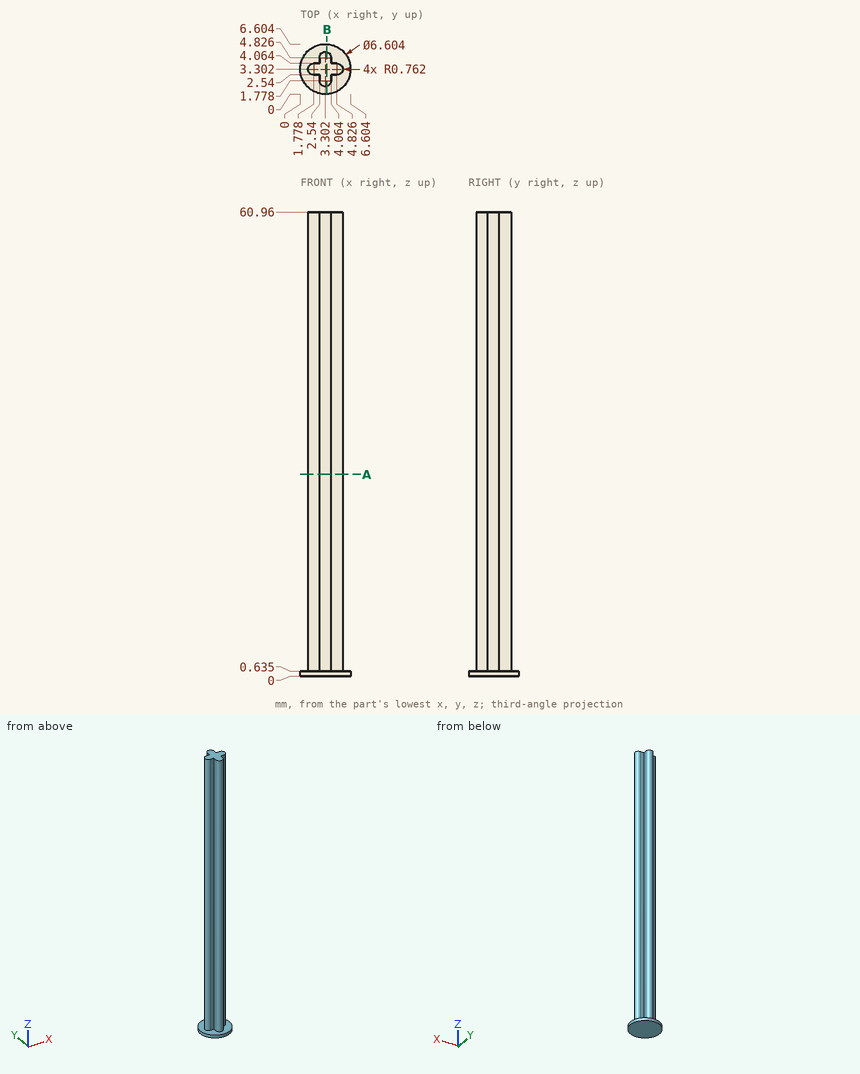
Input: dimensioned drawing with shaded views. Units: mm. Origin: part minimum x, y, z. Coordinates: 2 decimals unless noted, no trailing zeros. Loops run counter-clockwise (first coordinate to the right, second up) from the corner with the lowest first, then second, coordinate; pieces in that order, holes last. Notation, with made-up numbers: M 32,57.5 L 62,57.5 A24 cw 62,95.5 Z; hole C -6,66.5 d3. An arc over 180 degrees is marked long. Use a Markdown table: item, result. Add a question column.
1) Section A-A, the plane z = 26.5. Return the cut outline in (x, y), plus the area to 3 significant figures.
2) Pin query (flat end, axial travel): P1, Ø1.5, axis at y = 2, z = 33.5, coming from the -X side; P2, Ø3, axis at x = 2.5, z = 19, coming from the +Y side; P3, Ø0.6, axis at x = 2, z = 42, coming from the -Y side. Return the tip coordinate at first contact, or that it passes through.
3) Line query: L1, parallel to Z at x = 4.25, y = 0.5 (3 decimals); L2, parallel to Y at x = 2.25, z = 22. Output: solid intervals per line, ascending. Write a range as from..to.
4) Section B-B, the plane x = 3.5. Return the cut outline in (y, z) (3 decimals).
Answer below:
| question | item | result |
|---|---|---|
| 1 | outline | M 1.78,2.54 L 2.54,2.54 L 2.54,1.78 A0.76 ccw 4.06,1.78 L 4.06,2.54 L 4.83,2.54 A0.76 ccw 4.83,4.06 L 4.06,4.06 L 4.06,4.83 A0.76 ccw 2.54,4.83 L 2.54,4.06 L 1.78,4.06 A0.76 ccw Z |
| 1 | area | 10.6 mm2 |
| 2 | P1 | x = 1.25 |
| 2 | P2 | y = 5.59 |
| 2 | P3 | y = 2.54 |
| 3 | L1 | 0..0.635 |
| 3 | L2 | 2.54..4.06 |
| 4 | outline | M 0.006,0 L 6.598,0 L 6.598,0.635 L 5.562,0.635 L 5.562,60.96 L 1.042,60.96 L 1.042,0.635 L 0.006,0.635 Z |
